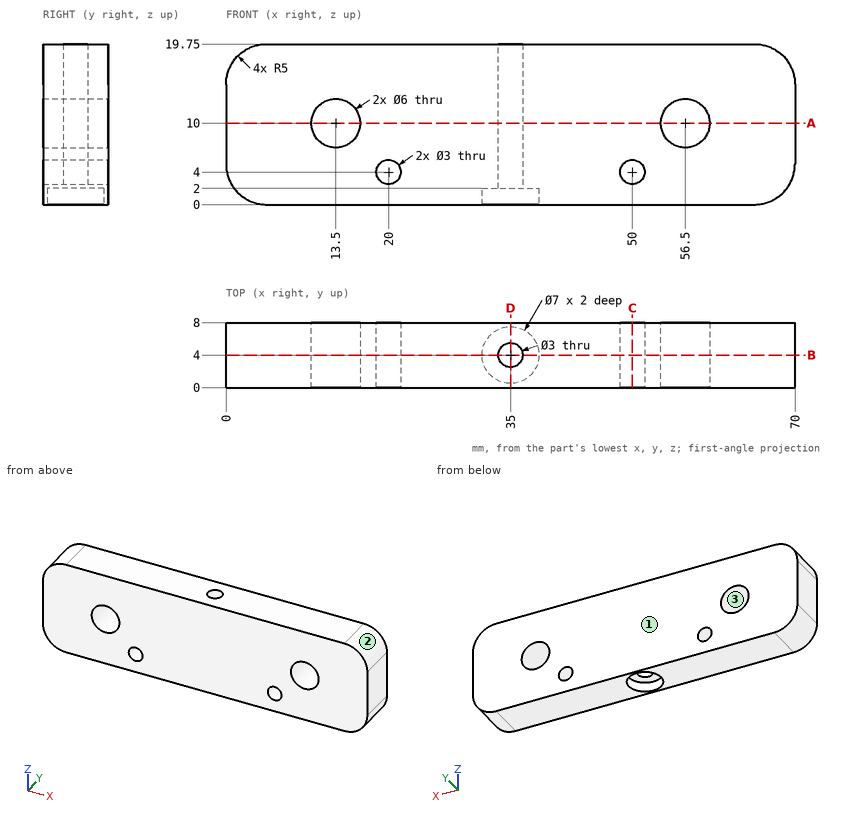
Could you check a few things on this drawing? It's one solid part, dimensions in mm from its lowest x, y, z. Coordinates: 2 decimals unless noted, no trailing zeros. Write each loop counter-clockwise with the first axis right and the second up, starting at its lowest first coordinate (ties: lowest second). Pieces come first, ordered by that corner, then holes.
Q1. Imagine slicing it at D-D, the plane x = 35. List the corners of the cut face in (y, z) for me.
Results found:
outline: (0, 0) - (0.5, 0) - (0.5, 2) - (2.5, 2) - (2.5, 19.75) - (0, 19.75) - close; (5.5, 2) - (7.5, 2) - (7.5, 0) - (8, 0) - (8, 19.75) - (5.5, 19.75) - close
Q2. Imagine slicing it at A-A, the plane z = 10. List the corners of the cut face in (x, y) for me.
Results found:
outline: (0, 0) - (10.5, 0) - (10.5, 8) - (0, 8) - close; (16.5, 0) - (53.5, 0) - (53.5, 8) - (16.5, 8) - close; (59.5, 0) - (70, 0) - (70, 8) - (59.5, 8) - close; hole circle Ø3 at (35, 4)
Q3. Imagine slicing it at C-C, the plane x = 50. List the corners of the cut face in (y, z) for me, plus the area to 3 significant figures.
Results found:
outline: (0, 0) - (8, 0) - (8, 2.5) - (0, 2.5) - close; (0, 5.5) - (8, 5.5) - (8, 19.75) - (0, 19.75) - close
area: 134 mm2
Q4. Please list where these lines run through material, in increasing order: L1, parallel to Z at x = 56.5, y = 3; L2, parallel to Y at x = 35, z = 1.25; L3, parallel to X at y = 6.75, z = 10.
Results found:
L1: z = 0 to 7, 13 to 19.75
L2: y = 0 to 0.5, 7.5 to 8
L3: x = 0 to 10.5, 16.5 to 53.5, 59.5 to 70
Q5. For P1, Ø2.5, axis at x = 50, z = 4, coming from the -Y side; P2, Ø2, axis at x = 34.5, y = 5.5, coming from the -Z side, each with a flat end and sliding along its axis, tell me the tip position at first contact or that it passes through.
Results found:
P1: passes through
P2: stops at z = 2
Q6. If we mould it in two halves opening along Z, with no side actions, what happens to the marked faces 1, 2 and 3? For each: +Z half, -Z half, draft (parallel to the pull), parting line (faces both ways), or undercut.
Results found:
face 1: draft
face 2: +Z half
face 3: undercut
Q7. Imagine slicing it at B-B, the plane y = 4. List the corners of the cut face in (x, z) for me.
Results found:
outline: (0, 5) arc R5 ccw to (5, 0) - (31.5, 0) - (31.5, 2) - (33.5, 2) - (33.5, 19.75) - (5, 19.75) arc R5 ccw to (0, 14.75) - close; (36.5, 2) - (38.5, 2) - (38.5, 0) - (65, 0) arc R5 ccw to (70, 5) - (70, 14.75) arc R5 ccw to (65, 19.75) - (36.5, 19.75) - close; hole circle Ø6 at (13.5, 10); hole circle Ø3 at (20, 4); hole circle Ø3 at (50, 4); hole circle Ø6 at (56.5, 10)
